Study the drawing (mm; zero at the part's minimum x, y, z) and answer. Give positions to 0.01 mm unless a question says otherwise; leave off trailing zeros. Write each loop counter-clockwise with the first axis right and the second up, starting at its lowest first coordinate (ties: lowest second). Pieces come first, ordered by that corner, then holes.
1) Given pin 1 Ø4 at (y, z) = (34, 125) entering from +X; pin 2 Ø1.5 at (x, y) = (3.5, 41) entering from +Z; pin 3 Ø3 at (x, z) = (2, 156.5) entering from -Y; pin 4 Ø1.8 at (x, z) = (4, 3.5) entering from +Y, each flat-ended and moving along its own axis, determine where each tip first touches the part or whether it passes through.
2) Find section C-C (x = 3.35). Determine the outline of the cut face in (y, z).
3) Find section A-A (z = 41.9). Determine the outline of the cut face in (x, y).
4) Straight lines are drawn through the part: probe 1 along Y at (x, z) = (1.6, 41.9); probe 2 along Z at (x, y) = (4.75, 34); probe 3 along Z at (x, y) = (3.3, 13.5). For each, find the intervals that lie inside material, in ascending order.
5) Find section B-B (y = 40). Determine the outline of the cut face in (x, z).
6) Find section D-D (z = 77). Determine the outline of the cut face in (x, y).
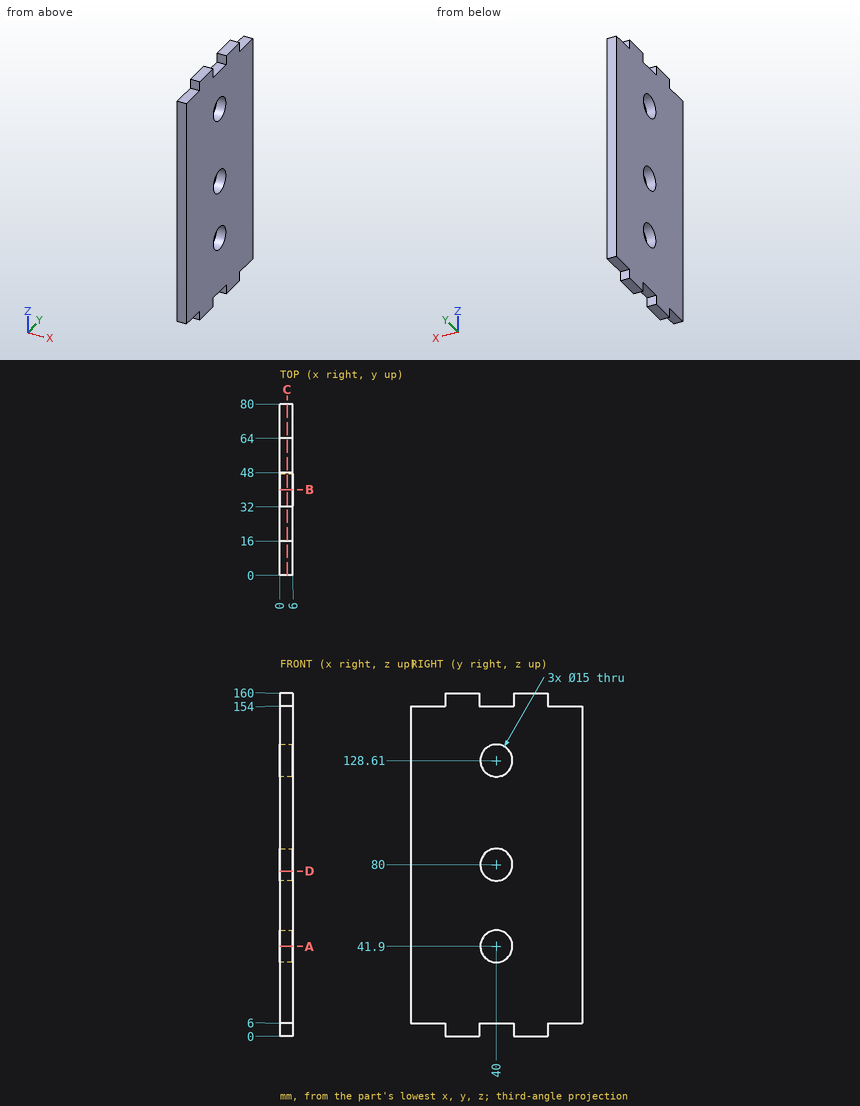
Results:
1. pin 1: stops at x = 6
1. pin 2: stops at z = 154
1. pin 3: stops at y = 16
1. pin 4: stops at y = 64
2. outline: (0, 6) - (16, 6) - (16, 0) - (32, 0) - (32, 6) - (48, 6) - (48, 0) - (64, 0) - (64, 6) - (80, 6) - (80, 154) - (64, 154) - (64, 160) - (48, 160) - (48, 154) - (32, 154) - (32, 160) - (16, 160) - (16, 154) - (0, 154) - close; hole circle Ø15 at (40, 41.9); hole circle Ø15 at (40, 80); hole circle Ø15 at (40, 128.61)
3. outline: (0, 0) - (6, 0) - (6, 32.5) - (0, 32.5) - close; (0, 47.5) - (6, 47.5) - (6, 80) - (0, 80) - close
4. probe 1: y = 0 to 32.5, 47.5 to 80
4. probe 2: z = 6 to 37.4, 46.4 to 75.5, 84.5 to 124.11, 133.11 to 154
4. probe 3: z = 6 to 154
5. outline: (0, 6) - (6, 6) - (6, 34.4) - (0, 34.4) - close; (0, 49.4) - (6, 49.4) - (6, 72.5) - (0, 72.5) - close; (0, 87.5) - (6, 87.5) - (6, 121.11) - (0, 121.11) - close; (0, 136.11) - (6, 136.11) - (6, 154) - (0, 154) - close
6. outline: (0, 0) - (6, 0) - (6, 33.13) - (0, 33.13) - close; (0, 46.87) - (6, 46.87) - (6, 80) - (0, 80) - close
